The listing builds one solid part. Answer for the finished solid, in the listing's coordinates (mm). Face numbers are marked on the shaded views. Round coordinates to 2 decimals unless told otherwise and drop trailing zeros. Loops run counter-clockwise (first coordinate to the right, second up) from the corner with the lowest first, then second, coordinate; pieces in that order, holes last. Notation, with made-up numbers: (-24, 30) -> (-14, 30) arc R7 ccw to (-14, 35) -> close; hole circle Ø4 at (10.25, 12). An arc over 180 degrees is marked (long way). Answer in a Markdown table with one row per item. Add a question column.
```python
from build123d import *

# Parameters (mm, degrees)
BOSS_EXTRUDE1_DEPTH = 6.35
SKETCH2_R           = 1.35
SKETCH2_R_2         = 1.385
CUT_EXTRUDE1_DEPTH  = 38.116505762
SKETCH3_W           = 63.5
SKETCH3_H           = 88.9
SKETCH3_W_2         = 38.321076004
SKETCH3_H_2         = 47.237540142
BOSS_EXTRUDE2_DEPTH = 6.35
SKETCH5_W           = 27.94
SKETCH5_H           = 55.88
CUT_EXTRUDE3_DEPTH  = 61.153053743
SKETCH6_R           = 3.175
CUT_EXTRUDE4_DEPTH  = 61.153053743
FILLET2_R           = 7.62
SKETCH7_W           = 41.724968974
SKETCH7_H           = 57.858351452
BOSS_EXTRUDE3_DEPTH = 6.35
SKETCH8_R           = 14.2875
CUT_EXTRUDE5_DEPTH  = 6.35


with BuildPart() as part:
    # Sketch1 → Boss-Extrude1 (new body)
    with BuildSketch(Plane.XY):
        with BuildLine():
            Line((-19.69889026, 23.2987845), (-14.850045261, 29.75147823))
            ThreePointArc((-14.850045261, 29.75147823), (-14.144755454, 30.339267512), (-13.251155001, 30.55))
            Line((-13.251155001, 30.55), (13.251155001, 30.55))
            ThreePointArc((13.251155001, 30.55), (14.144755454, 30.339267512), (14.850045261, 29.75147823))
            Line((14.850045261, 29.75147823), (19.69889026, 23.2987845))
            ThreePointArc((19.69889026, 23.2987845), (19.997074131, 22.730638521), (20.1, 22.09730627))
            Line((20.1, 22.09730627), (20.1, -22.09730627))
            ThreePointArc((20.1, -22.09730627), (19.997074131, -22.730638521), (19.69889026, -23.2987845))
            Line((19.69889026, -23.2987845), (14.850045261, -29.75147823))
            ThreePointArc((14.850045261, -29.75147823), (14.144755454, -30.339267512), (13.251155001, -30.55))
            Line((13.251155001, -30.55), (-13.251155001, -30.55))
            ThreePointArc((-13.251155001, -30.55), (-14.144755454, -30.339267512), (-14.850045261, -29.75147823))
            Line((-14.850045261, -29.75147823), (-19.69889026, -23.2987845))
            ThreePointArc((-19.69889026, -23.2987845), (-19.997074131, -22.730638521), (-20.1, -22.09730627))
            Line((-20.1, -22.09730627), (-20.1, 22.09730627))
            ThreePointArc((-20.1, 22.09730627), (-19.997074131, 22.730638521), (-19.69889026, 23.2987845))
        make_face()
    extrude(amount=-BOSS_EXTRUDE1_DEPTH)

    # Sketch2 → Cut-Extrude1 (cut, through all)
    with BuildSketch(Plane(origin=(0, 0, -6.35), x_dir=(-1, 0, 0), z_dir=(0, 0, -1))):
        with Locations((17.3, 21.9487845)):
            Circle(SKETCH2_R)
        with Locations((17.3, -0.0512155)):
            Circle(SKETCH2_R)
        with Locations((17.3, -22.0512155)):
            Circle(SKETCH2_R)
        with Locations((11, -27.75)):
            Circle(SKETCH2_R_2)
        with Locations(Location((-11, -27.75, 0), (0, 0, 180))):
            Circle(SKETCH2_R_2)
        with Locations(Location((-17.3, -22.0512155, 0), (0, 0, 180))):
            Circle(SKETCH2_R)
        with Locations(Location((-17.3, -0.0512155, 0), (0, 0, 180))):
            Circle(SKETCH2_R)
        with Locations(Location((-17.3, 21.9487845, 0), (0, 0, 180))):
            Circle(SKETCH2_R)
    extrude(amount=-CUT_EXTRUDE1_DEPTH, mode=Mode.SUBTRACT)

    # Sketch3 → Boss-Extrude2 (add)
    with BuildSketch(Plane(origin=(0, 0, -6.35), x_dir=(-1, 0, 0), z_dir=(0, 0, -1))):
        with Locations((0, -6.2452155)):
            Rectangle(SKETCH3_W, SKETCH3_H)
        Rectangle(SKETCH3_W_2, SKETCH3_H_2, mode=Mode.SUBTRACT)
    extrude(amount=-BOSS_EXTRUDE2_DEPTH)

    # Sketch5 → Cut-Extrude3 (cut, through all)
    with BuildSketch(Plane.XY):
        with Locations((0, 3.0087845)):
            Rectangle(SKETCH5_W, SKETCH5_H)
    extrude(amount=-CUT_EXTRUDE3_DEPTH, mode=Mode.SUBTRACT)

    # Sketch6 → Cut-Extrude4 (cut, through all)
    with BuildSketch(Plane(origin=(0, 0, -6.35), x_dir=(-1, 0, 0), z_dir=(0, 0, -1))):
        with Locations((25.4, 31.8547845)):
            Circle(SKETCH6_R)
        with Locations((-25.4, 31.8547845)):
            Circle(SKETCH6_R)
        with Locations((-25.4, -36.7252155)):
            Circle(SKETCH6_R)
        with Locations((25.4, -36.7252155)):
            Circle(SKETCH6_R)
    extrude(amount=-CUT_EXTRUDE4_DEPTH, mode=Mode.SUBTRACT)

    # Fillet2
    fillet2_edges = [part.edges().sort_by_distance(p)[0] for p in [
        (-31.75, 38.2047845, -3.175),
        (-31.75, -50.6952155, -3.175),
        (31.75, -50.6952155, -3.175),
        (31.75, 38.2047845, -3.175),
    ]]
    fillet(fillet2_edges, radius=FILLET2_R)

    # Sketch7 → Boss-Extrude3 (add)
    with BuildSketch(Plane(origin=(0, 0, -6.35), x_dir=(-1, 0, 0), z_dir=(0, 0, -1))):
        with Locations((0, 3.16744248)):
            Rectangle(SKETCH7_W, SKETCH7_H)
    extrude(amount=-BOSS_EXTRUDE3_DEPTH)

    # Sketch8 → Cut-Extrude5 (cut)
    with BuildSketch(Plane(origin=(0, 0, -6.35), x_dir=(-1, 0, 0), z_dir=(0, 0, -1))):
        with Locations((0, 17.8847845)):
            Circle(SKETCH8_R)
    extrude(amount=-CUT_EXTRUDE5_DEPTH, mode=Mode.SUBTRACT)


solid = part.part
```
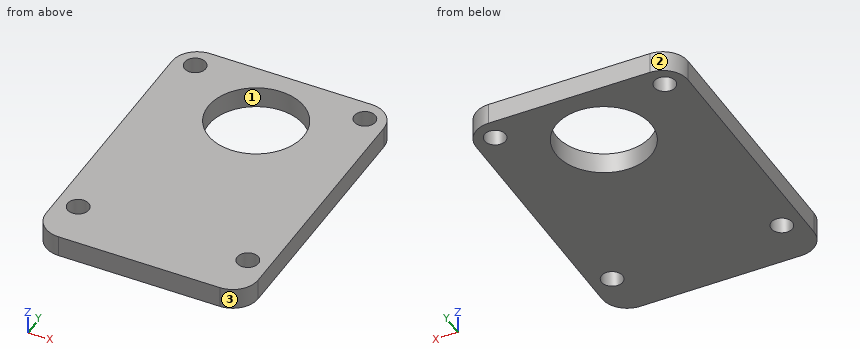
Item 1: Section B-B, the plane z = -3.25 is taken. Give the number of separate pieces and of enclosed holes in the cut face, and give its area (3 significant figures).
Item 2: The mould has two halves that part along X. Classify the marked faces 1, 2 and 3: +X half, -X half, draft (parallel to the pull), parting line (faces both ways), or undercut.
Item 3: Section D-D, the plane x = 25.5 is taken. Write down the section's boundary in (y, z).
Item 4: Section C-C, the plane x = -25.4 is taken. Write down the section's boundary in (y, z).
Item 5: Section A-A, the plane x = 0 is taken. Write down the section's boundary in (y, z), and give its area (3 significant figures).
Item 6: Consider L1, parallel to X at y = -38, z = -1; L2, parallel to Y at x = -27, z = -4; L3, parallel to X at y = -39.5, z = -1.25. Determine where each line is inside the solid, lowest interval first. Write a range as from..to.
Here are the results:
| question | item | result |
|---|---|---|
| 1 | separate pieces | 1 |
| 1 | enclosed holes | 5 |
| 1 | area | 4,830 mm² |
| 2 | face 1 | undercut |
| 2 | face 2 | -X half |
| 2 | face 3 | +X half |
| 3 | outline | (-50.57, -6.35) -> (-39.9, -6.35) -> (-39.9, 0) -> (-50.57, 0) -> close; (-33.55, -6.35) -> (28.68, -6.35) -> (28.68, 0) -> (-33.55, 0) -> close; (35.03, -6.35) -> (38.08, -6.35) -> (38.08, 0) -> (35.03, 0) -> close |
| 4 | outline | (-50.59, -6.35) -> (-39.9, -6.35) -> (-39.9, 0) -> (-50.59, 0) -> close; (-33.55, -6.35) -> (28.68, -6.35) -> (28.68, 0) -> (-33.55, 0) -> close; (35.03, -6.35) -> (38.1, -6.35) -> (38.1, 0) -> (35.03, 0) -> close |
| 5 | outline | (-50.7, -6.35) -> (3.6, -6.35) -> (3.6, 0) -> (-50.7, 0) -> close; (32.17, -6.35) -> (38.2, -6.35) -> (38.2, 0) -> (32.17, 0) -> close |
| 5 | area | 383 mm² |
| 6 | L1 | x = -31.75..-28.31, -22.49..22.49, 28.31..31.75 |
| 6 | L2 | y = -50.13..-39.47, -33.98..29.11, 34.6..37.64 |
| 6 | L3 | x = -31.75..-26.94, -23.86..23.86, 26.94..31.75 |
